Can you work these out from the model? Positions are in its coordinate system, mm. Face numbers are marked on the shaded views. Coordinates: 2 decimals unless noted, no trailing zeros. Loops run counter-clockwise (first coordinate to the right, second up) from the corner with the lowest first, then second, coordinate; pieces in that order, holes last.
```python
from build123d import *

# Parameters (mm, degrees)
F2_R     = 3
F3_DEPTH = 63
F4_R     = 5
F5_DEPTH = 12
F6_W     = 2.5
F6_H     = 11.932325


with BuildPart() as f1:
    # F0 (on Front) → F1 (revolve)
    with BuildSketch(Plane.XZ):
        with BuildLine():
            ThreePointArc((-37.441203, 0), (-37.136928, -3.059921), (-36.236017, -6))
            Line((-36.236017, -6), (28.763983, -6))
            Line((28.763983, -6), (28.763983, 0))
            Line((28.763983, 0), (-37.441203, 0))
        make_face()
    revolve(axis=Axis((-4.33861, 0, 0), (-1, 0, 0)))

    # F2 (on face) → F3 (cut)
    with BuildSketch(Plane.YZ.offset(28.763983)):
        Circle(F2_R)
    extrude(amount=-F3_DEPTH, mode=Mode.SUBTRACT)

    # F4 (on face) → F5 (cut)
    with BuildSketch(Plane.YZ.offset(28.763983)):
        Circle(F4_R)
    extrude(amount=-F5_DEPTH, mode=Mode.SUBTRACT)

    # F6 (on Top) → F7 (revolve, cut)
    with BuildSketch(Plane.XY):
        with Locations((-24.986017, -5.966162)):
            Rectangle(F6_W, F6_H)
    revolve(axis=Axis((-26.236017, -5.966163, 0), (0, -1, 0)), mode=Mode.SUBTRACT)


solid = f1.part
```
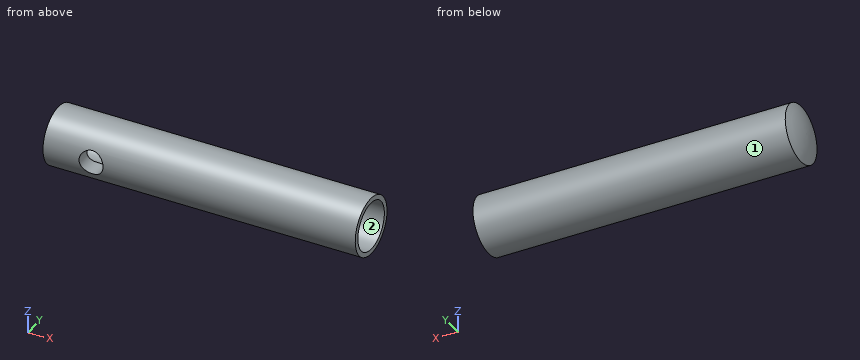
Item 1: Suppose I cut it at B-B, the plane x = -2. Please give me the cut outline in (y, z), plus the area to 3 significant figures.
Results are:
outline: circle Ø12 at (0, 0); hole circle Ø6 at (0, 0)
area: 84.8 mm2
Item 2: Suppose I cut it at A-A, the plane x = 21. Please give me the cut outline in (y, z).
Results are:
outline: circle Ø12 at (0, 0); hole circle Ø10 at (0, 0)
Item 3: I'm going to push flat-ended pins straight in: P1, Ø4, axis at x = -26.24, z = 0, coming from the -Y side; P2, Ø1.8, axis at y = -1.5, z = 0, coming from the +X side; P3, Ø2, axis at x = -6.5, y = -3.5, coming from the +Z side. Where does each tip first touch, or does it pass through?
Results are:
P1: stops at y = 2.24
P2: stops at x = -34.24
P3: stops at z = 5.45
Item 4: Suppose I cut it at C-C, the plane x = -27.5. Please give me the cut outline in (y, z).
Results are:
outline: (-5.6, -2.16) arc R6 ccw (long way) to (-5.6, 2.16) - (-2.09, 2.16) arc R3 cw (long way) to (-2.09, -2.16) - close
Item 5: We'd pull the mould along Z, two halves only. Please class the marked faces 1 and 2: +Z half, -Z half, draft (parallel to the pull), parting line (faces both ways), or undercut.
Results are:
face 1: parting line
face 2: undercut
Item 6: I need wall thicknesses on line 1 along Z through (x, y) = (3, -0.25); line 2 along Y through (x, z) = (5, 0); line 3 along Z through (x, y) = (-28, -2.25). Which ranges of each line are inside material? Lowest first, please.
Results are:
line 1: z = -5.99 to -2.99, 2.99 to 5.99
line 2: y = -6 to -3, 3 to 6
line 3: z = -5.56 to -1.98, 1.98 to 5.56
